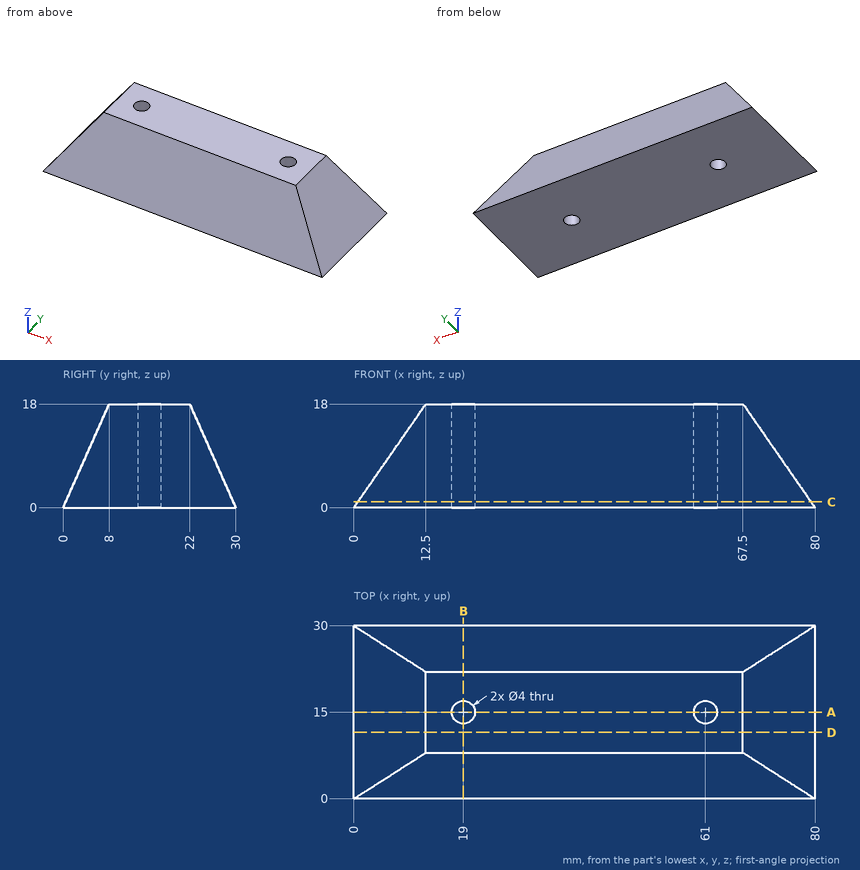
For this review, use the dimensioned drawing (mm, ordinates from the lowest corner) and the shaded views. Give positions to 0.01 mm unless a question says otherwise; leave off trailing zeros. Loops run counter-clockwise (first coordinate to the right, second up) from the corner with the lowest first, then second, coordinate; pieces in that order, holes last.
Item 1: Take a section at C-C, the plane z = 1. State the section outline as (x, y) points, and give its area (3 significant figures).
Item 2: Take a section at D-D, the plane y = 11.5. State the section outline as (x, z) points, and give its area (4 significant figures).
Item 3: Take a section at B-B, the plane x = 19. State the section outline as (y, z) points, and give its area (3 significant figures).
Item 4: Take a section at A-A, the plane y = 15. State the section outline as (x, z) points.
Item 5: For line 1 along X through (y, z) = (14, 4); line 2 along Y through (x, z) = (19, 4.25); line 3 along Y through (x, z) = (61, 7.75), list the stretches that pass through material, from the lowest coordinate up.
Item 6: Insertion check: pin 1 (10 mm diameter, centred on x = 28.5, z = 16, fed in from -Y); pin 2 (6 mm diameter, centred on y = 12.5, z = 9.5, fed in from -X); pin 3 (4 mm diameter, centred on y = 18, z = 13, fed in from -X); pin 4 (6.5 mm diameter, centred on x = 19, y = 15, fed in from +Z). Each pin has a flat end and moves straight along its axis. Give the tip position at first contact, or say it passes through.
Calculated:
1. outline: (0.69, 0.44) - (79.31, 0.44) - (79.31, 29.56) - (0.69, 29.56) - close; hole circle Ø4 at (19, 15); hole circle Ø4 at (61, 15)
1. area: 2,260 mm2
2. outline: (0, 0) - (80, 0) - (67.5, 18) - (12.5, 18) - close
2. area: 1,215 mm2
3. outline: (0, 0) - (13, 0) - (13, 18) - (8, 18) - close; (17, 0) - (30, 0) - (22, 18) - (17, 18) - close
3. area: 324 mm2
4. outline: (0, 0) - (17, 0) - (17, 18) - (12.5, 18) - close; (21, 0) - (59, 0) - (59, 18) - (21, 18) - close; (63, 0) - (80, 0) - (67.5, 18) - (63, 18) - close
5. line 1: x = 2.78 to 17.27, 20.73 to 59.27, 62.73 to 77.22
5. line 2: y = 1.89 to 13, 17 to 28.11
5. line 3: y = 3.44 to 13, 17 to 26.56
6. pin 1: stops at y = 4.89
6. pin 2: stops at x = 4.51
6. pin 3: stops at x = 7.64
6. pin 4: stops at z = 18
